Geometry check sheet. Reference: drawing and pictorial views, mm from the part's lowest x, y, z. Coordinates: 2 decimals unless noted, no trailing zeros. Write each loop counter-clockwise with the first axis right and the second up, starting at its lowest first coordinate (ties: lowest second). Pieces come first, ordered by that corner, then holes. Notation, with made-up numbers: (83.25, 23.5) - (110.25, 23.5) arc R20 ccw to (110.25, 28.5) - close; hole circle Ø4 at (-32.75, 63.5). An arc over 180 degrees is marked (long way). Answer as CSV lines item,"result". Start each with the question number.
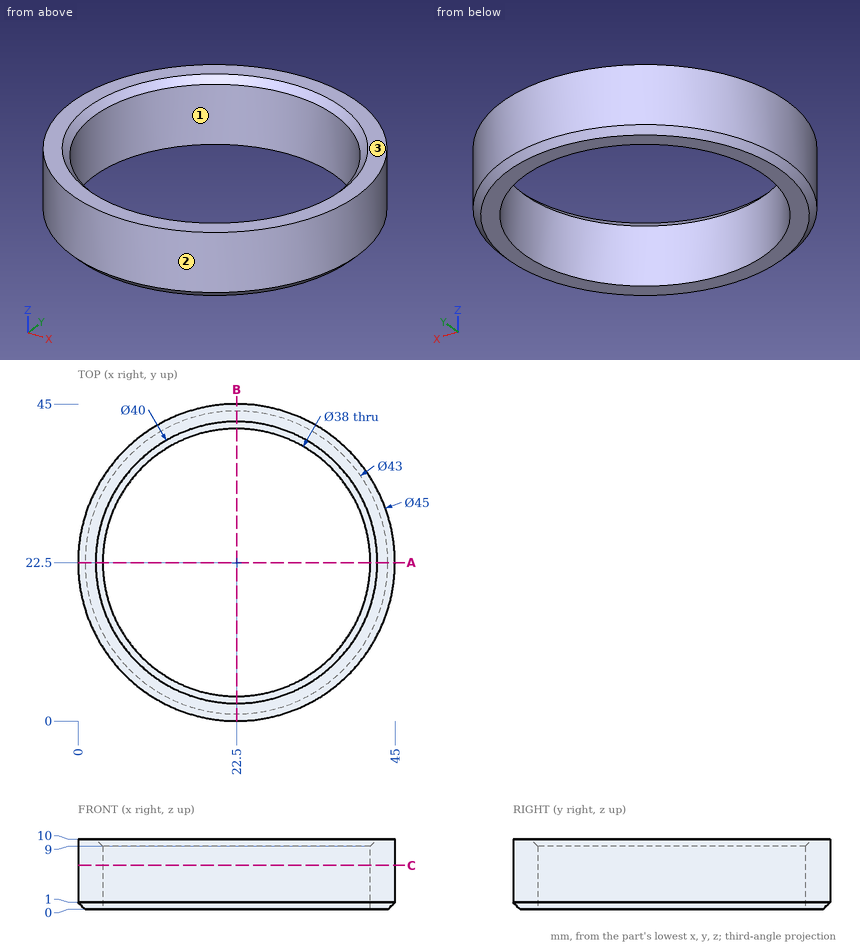
1. Scan lines: line 1 along Y through (x, z) = (22.5, 3); line 2 along X through (y, z) = (33.5, 9); line 3 along X through (y, z) = (23.5, 5.75). Record each from-to range of solid material in increasing order. Write a range as from..to.
2. Cross-section at A-A (y = 22.5). Record the cut outline in (x, z).
3. Draft check along Y on the marked faces 1, 2 and 3. Enter one of: pulls with the +Y half, pulls with the -Y half, needs draft (parallel to the pull), parting line crosses it, or undercut.
4. Cross-section at C-C (z = 6.25). Record the cut outline in (x, y), and give its area (3 significant figures).
5. Depth check by flat-ended pin: P1, Ø1, axis at y = 7.5, z = 3, coming from the +X side; P2, Ø4, axis at y = 28.5, z = 3.5, coming from the +X side; P3, Ø1.5, axis at x = 24.5, z = 1.5, coming from the -Y side. Enter the tip coordinate at first touch or a pass-through.
Completed:
1,line 1,"y = 0..3.5, 41.5..45"
1,line 2,"x = 2.87..7.01, 37.99..42.13"
1,line 3,"x = 0.02..3.53, 41.47..44.98"
2,outline,"(0, 1) - (1, 0) - (3.5, 0) - (3.5, 9) - (2.5, 10) - (0, 10) - close; (41.5, 0) - (44, 0) - (45, 1) - (45, 10) - (42.5, 10) - (41.5, 9) - close"
3,face 1,"undercut"
3,face 2,"parting line crosses it"
3,face 3,"needs draft"
4,outline,"circle Ø45 at (22.5, 22.5); hole circle Ø38 at (22.5, 22.5)"
4,area,"456 mm2"
5,P1,"stops at x = 39.7"
5,P2,"stops at x = 44.64"
5,P3,"stops at y = 0.03"
